from build123d import *

# Parameters (mm, degrees)
ESQUISSE1_R        = 12.5
BOSS_EXTRU_2_DEPTH = 2.9
CHANFREIN2_SIZE    = 0.25
CHANFREIN3_SIZE    = 0.25


with BuildPart() as part:
    # Esquisse1 → Boss.-Extru.2 (new body)
    with BuildSketch(Plane.XY):
        Circle(ESQUISSE1_R)
    extrude(amount=BOSS_EXTRU_2_DEPTH)

    # Chanfrein2
    chanfrein2_edges = [part.edges().sort_by_distance(p)[0] for p in [
        (-12.5, 0, 2.9),
    ]]
    chamfer(chanfrein2_edges, length=CHANFREIN2_SIZE)

    # Chanfrein3
    chanfrein3_edges = [part.edges().sort_by_distance(p)[0] for p in [
        (-12.5, 0, 0),
    ]]
    chamfer(chanfrein3_edges, length=CHANFREIN3_SIZE)


solid = part.part
Model file for the job. Use its own axes, mm. Round coordinates to 2 decimals unless told otherwise and drop trailing zeros. Order: outer loops, then holes, each group sorted by start corner. A loop starts at its lowest first (then second) coordinate and runs counter-clockwise, first axis right, second up.
(1) Pin check, flat tips, straight feed: pin 1 (1 mm diameter, centred on x = 5.5, z = 1.5, fed in from -Y); pin 2 (1.5 mm diameter, centred on x = -2, z = 0.5, fed in from -Y); pin 3 (1 mm diameter, centred on x = -5, z = 2.5, fed in from -Y). Stop position of each tip, or through.
(2) Band-saw the part on A-A (z = 1.4). List the corners of the cut face in (x, y), then the cut area to 3 significant figures.
(3) Drill centre lines: line 1 (Y direction, x = 2.5, z = 0.55); line 2 (X direction, y = 10.75, z = 1.5); line 3 (X direction, y = 7.75, z = 1). Where is each one in solid material? Low to high.
Verdict:
1. pin 1: stops at y = -11.46
1. pin 2: stops at y = -12.44
1. pin 3: stops at y = -11.66
2. outline: circle Ø25 at (0, 0)
2. area: 491 mm2
3. line 1: y = -12.25 to 12.25
3. line 2: x = -6.38 to 6.38
3. line 3: x = -9.81 to 9.81
